```python
from build123d import *

# Parameters (mm, degrees)
SKETCH1_W           = 165.1
SKETCH1_H           = 114.3
SKETCH1_W_2         = 152.4
SKETCH1_H_2         = 101.6
SKETCH1_H_3         = 12.7
BOSS_EXTRUDE1_DEPTH = 2.54


with BuildPart() as part:
    # Sketch1 → Boss-Extrude1 (new body)
    with BuildSketch(Plane(origin=(0, 0, 0), x_dir=(1, 0, 0), z_dir=(0, 1, 0))):
        Rectangle(SKETCH1_W, SKETCH1_H)
        Rectangle(SKETCH1_W_2, SKETCH1_H_2, mode=Mode.SUBTRACT)
        Rectangle(SKETCH1_W_2, SKETCH1_H_3)
    extrude(amount=BOSS_EXTRUDE1_DEPTH)


solid = part.part
```
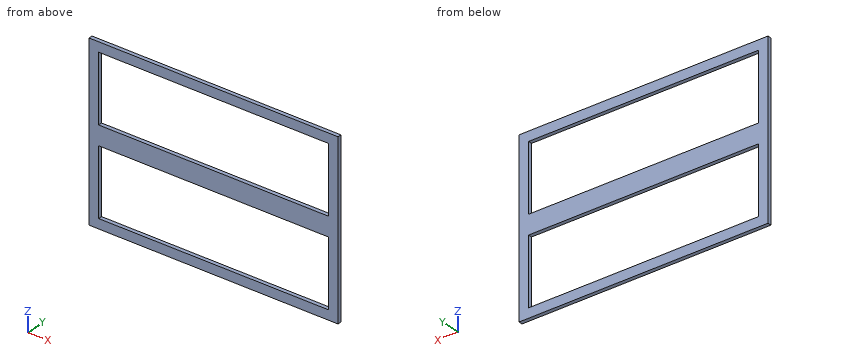
Design review of the part built by this model. Coordinates are the model's own, in mm. Coordinates: 2 decimals unless noted, no trailing zeros. Order: outer loops, then holes, each group sorted by start corner. A loop starts at its lowest first (then second) coordinate and runs counter-clockwise, first axis right, second up. Notation, with made-up numbers: (-17.5, -22.75) - (-1.5, -22.75) arc R19 cw to (-1.5, -15.75) - close; hole circle Ø7 at (38.25, 32). An arc over 180 degrees is marked (long way). One line per question, with ' | ' between items.
Q1. Consider section C-C, the plane z = 28. Give the boundary of the cut face in (x, y), then the cut area to 3 significant figures.
Answer key:
outline: (-82.55, 0) - (-76.2, 0) - (-76.2, 2.54) - (-82.55, 2.54) - close; (76.2, 0) - (82.55, 0) - (82.55, 2.54) - (76.2, 2.54) - close | area: 32.3 mm2
Q2. Consider section A-A, the plane x = 54. Give the boundary of the cut face in (y, z), then the cut area to 3 significant figures.
Answer key:
outline: (0, -57.15) - (2.54, -57.15) - (2.54, -50.8) - (0, -50.8) - close; (0, -6.35) - (2.54, -6.35) - (2.54, 6.35) - (0, 6.35) - close; (0, 50.8) - (2.54, 50.8) - (2.54, 57.15) - (0, 57.15) - close | area: 64.5 mm2
Q3. To check wall thickness, follow line 1 along Z through (x, y) = (-1.5, 0.7); line 2 along X through (y, z) = (1, 17). State the ranges of each line that lie inside material, in increasing order.
Answer key:
line 1: z = -57.15 to -50.8, -6.35 to 6.35, 50.8 to 57.15 | line 2: x = -82.55 to -76.2, 76.2 to 82.55
Q4. Consider section B-B, the plane y = 0.4. Give the boundary of the cut face in (x, z).
Answer key:
outline: (-82.55, -57.15) - (82.55, -57.15) - (82.55, 57.15) - (-82.55, 57.15) - close; hole (-76.2, -50.8) - (76.2, -50.8) - (76.2, -6.35) - (-76.2, -6.35) - close; hole (-76.2, 6.35) - (76.2, 6.35) - (76.2, 50.8) - (-76.2, 50.8) - close
